from build123d import *

# Parameters (mm, degrees)
SKETCH18_R          = 3.175
SKETCH18_R_2        = 6.35
SKETCH18_R_3        = 2.5019
BOSS_EXTRUDE4_DEPTH = 6.35
CHAMFER1_SIZE       = 2.54
SKETCH19_R          = 6.0325
CUT_EXTRUDE1_DEPTH  = 43.434
SKETCH20_W          = 20
SKETCH20_H          = 6.35
BOSS_EXTRUDE5_DEPTH = 20.32
FILLET1_R           = 2.54


with BuildPart() as part:
    # Sketch18 → Boss-Extrude4 (new body)
    with BuildSketch(Plane.XY):
        with BuildLine():
            Line((0, 0), (-265.604745697, 0))
            ThreePointArc((-265.604745697, 0), (-298.882523776, 76.131915965), (-307.699061234, 158.75))
            Line((-307.699061234, 158.75), (-307.699061234, 165.1))
            ThreePointArc((-307.699061234, 165.1), (-305.839189294, 169.590128061), (-301.349061234, 171.45))
            Line((-301.349061234, 171.45), (-231.499061234, 171.45))
            Line((-231.499061234, 171.45), (-159.473782125, 158.75))
            Line((-159.473782125, 158.75), (-28.014368889, 158.75))
            ThreePointArc((-28.014368889, 158.75), (-23.851207857, 157.194850386), (-21.727208485, 153.291130779))
            Line((-21.727208485, 153.291130779), (0, 0))
        make_face()
        with Locations((-11.423473622, 24.034728138)):
            Circle(SKETCH18_R, mode=Mode.SUBTRACT)
        with Locations((-27.253356194, 124.406511892)):
            Circle(SKETCH18_R, mode=Mode.SUBTRACT)
        with Locations((-35.200938766, 146.05)):
            Circle(SKETCH18_R_2, mode=Mode.SUBTRACT)
        with Locations((-301.900938766, 146.05)):
            Circle(SKETCH18_R, mode=Mode.SUBTRACT)
        with Locations((-301.569673588, 132.761391752)):
            Circle(SKETCH18_R, mode=Mode.SUBTRACT)
        with Locations((-300.579872803, 119.537524267)):
            Circle(SKETCH18_R, mode=Mode.SUBTRACT)
        with Locations((-298.943543444, 106.442822899)):
            Circle(SKETCH18_R, mode=Mode.SUBTRACT)
        with Locations((-239.568937637, 24.034728138)):
            Circle(SKETCH18_R, mode=Mode.SUBTRACT)
        with Locations((-286.962142025, 164.850708953)):
            Circle(SKETCH18_R, mode=Mode.SUBTRACT)
        with Locations((-165.1, 146.05)):
            Circle(SKETCH18_R_3, mode=Mode.SUBTRACT)
        with Locations((-143.102954744, 107.95)):
            Circle(SKETCH18_R_3, mode=Mode.SUBTRACT)
        with Locations((-187.097045256, 107.95)):
            Circle(SKETCH18_R_3, mode=Mode.SUBTRACT)
    extrude(amount=BOSS_EXTRUDE4_DEPTH)

    # Chamfer1
    chamfer1_edges = [part.edges().sort_by_distance(p)[0] for p in [
        (-14.598473622, 24.034728138, 6.35),
        (-30.428356194, 124.406511892, 6.35),
        (-242.743937637, 24.034728138, 6.35),
        (-290.137142025, 164.850708953, 6.35),
    ]]
    chamfer(chamfer1_edges, length=CHAMFER1_SIZE)

    # Sketch19 → Cut-Extrude1 (cut)
    with BuildSketch(Plane(origin=(0, 0, 0), x_dir=(-1, 0, 0), z_dir=(0, 0, -1))):
        with Locations((112.843509564, 96.674296134)):
            Circle(SKETCH19_R)
    extrude(amount=-CUT_EXTRUDE1_DEPTH, mode=Mode.SUBTRACT)

    # Sketch20 → Boss-Extrude5 (add)
    with BuildSketch(Plane.XZ):
        with Locations((-255.604745697, 3.175)):
            Rectangle(SKETCH20_W, SKETCH20_H)
        with Locations((-57.384832148, 3.175)):
            Rectangle(SKETCH20_W, SKETCH20_H)
    extrude(amount=BOSS_EXTRUDE5_DEPTH)

    # Fillet1
    fillet1_edges = [part.edges().sort_by_distance(p)[0] for p in [
        (-265.604745697, -20.32, 3.175),
        (-245.604745697, -20.32, 3.175),
        (-47.384832148, -20.32, 3.175),
        (-67.384832148, -20.32, 3.175),
    ]]
    fillet(fillet1_edges, radius=FILLET1_R)


solid = part.part
Design review of the part built by this model. Coordinates are the model's own, in mm. A direction names the side the tool comes from. Coordinates: 2 decimals unless noted, no trailing zeros. Loops run counter-clockwise (first coordinate to the right, second up) from the corner with the lowest first, then second, coordinate; pieces in that order, holes last. Notation, with made-up numbers: M 32.25,19 L 53.25,19 A10 cw 53.25,37 Z; hole C -11.5,82 d7. An arc over 180 degrees is marked long. Use one line per item in the form item = value.
(1) Draft analysis for pull direction X (two halves, no side actions). For faces 1 (the face through (-156, 77, 0)), 2 (the face through (-47.385, -9, 3)), 3 (the face through (-298.541, 133.715, 3.131)), state which applies: pulls with the +X half, pulls with the -X half, needs draft (parallel to the pull), parting line crosses it, or undercut.
Return value:
face_1 = needs draft
face_2 = pulls with the +X half
face_3 = undercut
(2) Consider section C-C (y = 8). Write out the cut boundary in (x, z), and give its area (3 significant figures).
Return value:
outline = M -270.49,0 L -1.13,0 L -1.13,6.35 L -270.49,6.35 Z
area = 1,710 mm2
(3) For line 1 along Y through (x, z) = (-30.5, 4.5); line 2 along X through (y, z) = (108.5, 0.75); line 3 along X through (y, z) = (-2, 4.25), list the stretches that pass through material, from the lowest coordinate up. Write a range as from..to.
Return value:
line_1 = 0..122.31, 126.5..141.78, 150.32..158.75
line_2 = -305.4..-301.36, -296.53..-189.54, -184.66..-145.54, -140.66..-15.38
line_3 = -265.6..-245.6, -67.38..-47.38
(4) For faces 4 (the face through (-265.605, -9, 3)), 5 (the face through (-95, 158.75, 3)), 6 (the face through (-307.699, 162, 3)), list the 3-axis set-ups (+Z, -Z, +X, -X, +Y, -Y) from which the entire face can be reached by the end or side of a thin tool; tool diameter is ignored.
Return value:
face_4 = +Z, -Z, -X, -Y
face_5 = +Z, -Z, +X, +Y
face_6 = +Z, -Z, -X, +Y
(5) Consider section B-B (x = -219). Write out the cut boundary in (y, z).
Return value:
outline = M 0,0 L 169.25,0 L 169.25,6.35 L 0,6.35 Z
(6) Clearance check with flat-ended pins moving along their axes: P1, Ø7.5, axis at x = -239.57, y = 24.03, coming from the +Z side; P2, Ø1.5, axis at x = -69, z = 1.5, coming from the +Y side; P3, Ø3, axis at x = -131.5, z = 4.5, coming from the -Y side; P4, Ø5.5, axis at x = -301.57, y = 132.76, coming from the +Z side. State where each tip first meets the part, or that it passes through.
Return value:
P1 = 4.39
P2 = 158.75
P3 = 0
P4 = through
(7) Consider section A-A (z = 5). Give the number of separate pieces and of enclosed holes in the cut face, and give its area (3 significant figures).
Return value:
separate_pieces = 1
enclosed_holes = 13
area = 46,700 mm2
